Can you work these out from the drawing? Everything is in mm from the part's minimum corner. Coordinates: 2 decimals unless noted, no trailing zeros. Order: outer loops, then holes, each group sorted by start corner. A loop starts at its lowest first (then second) coordinate and runs counter-clockwise, first axis right, second up. Notation, with made-up numbers: M -1.75,-23.5 L 3.25,-23.5 A15 ccw 3.25,-9.5 Z; hole C 61,25.25 d2. An arc over 180 degrees is marked long. Answer as a JSON object with one key per item and string values.
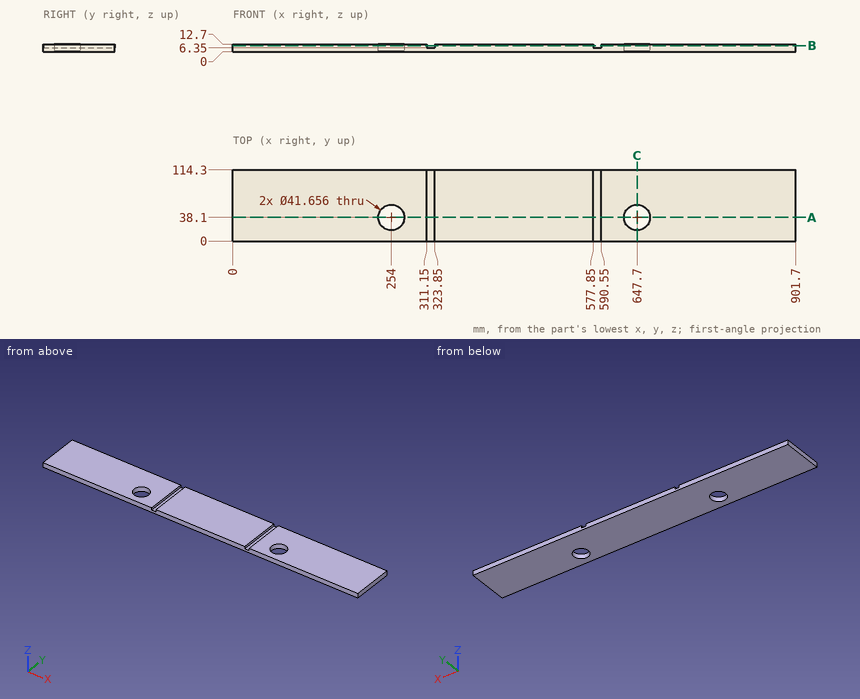
Item 1: I want a section at B-B, the plane z = 10.25. Write out the boundary of the cut face in (x, y).
Answers follow:
{"outline": "M 0,0 L 311.15,0 L 311.15,114.3 L 0,114.3 Z; M 323.85,0 L 577.85,0 L 577.85,114.3 L 323.85,114.3 Z; M 590.55,0 L 901.7,0 L 901.7,114.3 L 590.55,114.3 Z; hole C 254,38.1 d41.66; hole C 647.7,38.1 d41.66"}
Item 2: Please list where these lines run through material, in increasing order: line 1 (X direction, y = 95, z = 10.25); line 2 (Y direction, x = 254, z = 6); line 3 (X direction, y = 24.5, z = 11).
Answers follow:
{"line 1": "x = 0 to 311.15, 323.85 to 577.85, 590.55 to 901.7", "line 2": "y = 0 to 17.27, 58.93 to 114.3", "line 3": "x = 0 to 238.23, 269.77 to 311.15, 323.85 to 577.85, 590.55 to 631.93, 663.47 to 901.7"}
Item 3: I want a section at A-A, the plane y = 38.1. Write out the boundary of the cut face in (x, z).
Answers follow:
{"outline": "M 0,0 L 233.17,0 L 233.17,12.7 L 0,12.7 Z; M 274.83,0 L 626.87,0 L 626.87,12.7 L 590.55,12.7 L 590.55,6.35 L 577.85,6.35 L 577.85,12.7 L 323.85,12.7 L 323.85,6.35 L 311.15,6.35 L 311.15,12.7 L 274.83,12.7 Z; M 668.53,0 L 901.7,0 L 901.7,12.7 L 668.53,12.7 Z"}
Item 4: I want a section at C-C, the plane x = 647.7. Write out the boundary of the cut face in (y, z).
Answers follow:
{"outline": "M 0,0 L 17.27,0 L 17.27,12.7 L 0,12.7 Z; M 58.93,0 L 114.3,0 L 114.3,12.7 L 58.93,12.7 Z"}
Item 5: I'm going to push flat-ended pins straight in: pin 1 (14 mm diameter, centred on x = 319.5, y = 40.5, fed in from +Z); pin 2 (4 mm diameter, centred on x = 583, y = 79.5, fed in from +Z). Where does each tip first touch, or does it pass through?
Answers follow:
{"pin 1": "stops at z = 12.7", "pin 2": "stops at z = 6.35"}
